For this review, take the finished solid that the model builds, in its own axes (mm). Face numbers are marked on the shaded views. Give positions to 0.01 mm unless a question says otherwise; leave off trailing zeros. Loops run counter-clockwise (first coordinate to the right, second up) from the corner with the lowest first, then second, coordinate; pieces in that order, holes last. Notation, with made-up numbers: (20.5, 82) - (44.5, 82) arc R24 ccw to (44.5, 101) - close; hole circle Ø2 at (-17.75, 10). An arc over 180 degrees is marked (long way). Put each result on its own line as item: value.
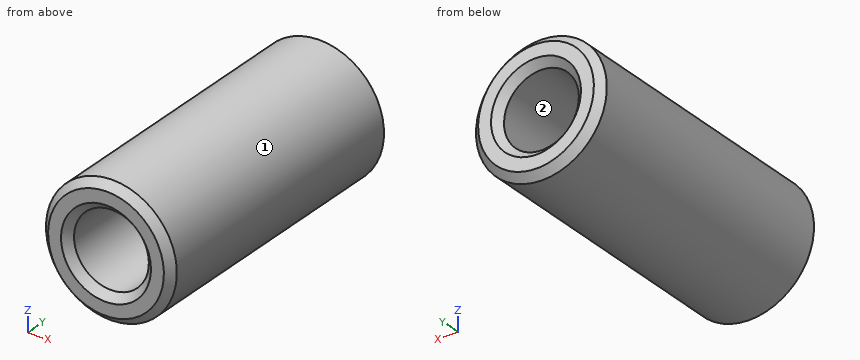
from build123d import *

# Parameters (mm, degrees)
CROQUIS1_R              = 6.5
CROQUIS1_R_2            = 3.715
SALIENTE_EXTRUIR1_DEPTH = 15
CHAFL_N1_SIZE           = 0.75


with BuildPart() as part:
    # Croquis1 → Saliente-Extruir1 (new, symmetric)
    with BuildSketch(Plane(origin=(0, 0, 0), x_dir=(1, 0, 0), z_dir=(0, 1, 0))):
        with Locations(Location((0, 0, 0), (0, 0, 270))):
            Circle(CROQUIS1_R)
        with Locations(Location((0, 0, 0), (0, 0, 270))):
            Circle(CROQUIS1_R_2, mode=Mode.SUBTRACT)
    extrude(amount=SALIENTE_EXTRUIR1_DEPTH, both=True)

    # Chaflán1
    chafl_n1_edges = [part.edges().sort_by_distance(p)[0] for p in [
        (0, -15, -6.5),
        (0, 15, -6.5),
        (0, -15, -3.715),
        (0, 15, -3.715),
    ]]
    chamfer(chafl_n1_edges, length=CHAFL_N1_SIZE)


solid = part.part
1) Insertion check: pin 1 Ø4 at (y, z) = (-6.5, 3) entering from -X; pin 2 Ø1.5 at (x, z) = (-2, 3) entering from +Y; pin 3 Ø4.5 at (x, z) = (0, 0) entering from +Y; pin 4 Ø1 at (x, y) = (-3.5, 0) entering from -Z. Each pin has a flat end and moves straight along its axis. Give the tip position at first contact, or say it passes through.
Geometry check:
pin 1: stops at x = -6.42
pin 2: stops at y = 14.89
pin 3: passes through
pin 4: stops at z = -5.77
2) Wall thickness on line 1 (X direction, y = 5.25, z = 0) (3 decimals); line 2 (Z direction, x = -3, y = 13.75); line 3 (Z direction, x = -2, y = 9.75): over which ranges is each line inside the solid? List them lowest first.
Geometry check:
line 1: x = -6.5 to -3.715, 3.715 to 6.5
line 2: z = -5.77 to -2.19, 2.19 to 5.77
line 3: z = -6.18 to -3.13, 3.13 to 6.18
3) Take a section at C-C on y = 6.5. State the section outline as (x, z) points (3 decimals).
Geometry check:
outline: circle Ø13 at (0, 0); hole circle Ø7.43 at (0, 0)
4) Draft analysis for pull direction Z (two halves, no side actions). For the marked faces 1 and 2, state which applies: pulls with the +Z half, pulls with the -Z half, needs draft (parallel to the pull), parting line crosses it, or undercut.
Geometry check:
face 1: parting line crosses it
face 2: undercut
5) Take a section at A-A on z = 0. State the section outline as (x, y) points (3 decimals).
Geometry check:
outline: (-6.5, -14.25) - (-5.75, -15) - (-4.465, -15) - (-3.715, -14.25) - (-3.715, 14.25) - (-4.465, 15) - (-5.75, 15) - (-6.5, 14.25) - close; (3.715, -14.25) - (4.465, -15) - (5.75, -15) - (6.5, -14.25) - (6.5, 14.25) - (5.75, 15) - (4.465, 15) - (3.715, 14.25) - close
6) Take a section at B-B on x = 0. State the section outline as (y, z) points (3 decimals), and give its area (3 significant figures).
Geometry check:
outline: (-15, -5.75) - (-14.25, -6.5) - (14.25, -6.5) - (15, -5.75) - (15, -4.465) - (14.25, -3.715) - (-14.25, -3.715) - (-15, -4.465) - close; (-15, 4.465) - (-14.25, 3.715) - (14.25, 3.715) - (15, 4.465) - (15, 5.75) - (14.25, 6.5) - (-14.25, 6.5) - (-15, 5.75) - close
area: 165 mm²
